```python
from build123d import *

# Parameters (mm, degrees)
ESQUISSE1_W             = 8
ESQUISSE1_H             = 48
BOSS_EXTRU_1_DEPTH      = 45
ESQUISSE28_R            = 7.95
ENL_V_MAT_EXTRU_1_DEPTH = 10
ESQUISSE29_R            = 8.1
ESQUISSE29_R_2          = 5.5
BOSS_EXTRU_2_DEPTH      = 3
ESQUISSE30_R            = 2
ENL_V_MAT_EXTRU_2_DEPTH = 15
ESQUISSE31_R            = 2
ENL_V_MAT_EXTRU_3_DEPTH = 15


with BuildPart() as part:
    # Esquisse1 → Boss.-Extru.1 (new body)
    with BuildSketch(Plane(origin=(0, 0, 0), x_dir=(1, 0, 0), z_dir=(0, 1, 0))):
        with Locations((4, 24)):
            Rectangle(ESQUISSE1_W, ESQUISSE1_H)
    extrude(amount=BOSS_EXTRU_1_DEPTH)

    # Esquisse28 → Enl_v. mat.-Extru.1 (cut)
    with BuildSketch(Plane(origin=(8, 0, 0), x_dir=(0, 0, -1), z_dir=(1, 0, 0))):
        with Locations((24, 18)):
            Circle(ESQUISSE28_R)
    extrude(amount=-ENL_V_MAT_EXTRU_1_DEPTH, mode=Mode.SUBTRACT)

    # Esquisse29 → Boss.-Extru.2 (add)
    with BuildSketch(Plane.ZY):
        with Locations((-24, 18)):
            Circle(ESQUISSE29_R)
        with Locations((-24, 18)):
            Circle(ESQUISSE29_R_2, mode=Mode.SUBTRACT)
    extrude(amount=-BOSS_EXTRU_2_DEPTH)

    # Esquisse30 → Enl_v. mat.-Extru.2 (cut)
    with BuildSketch(Plane.XZ):
        with Locations((4, -44)):
            Circle(ESQUISSE30_R)
        with Locations((4, -4)):
            Circle(ESQUISSE30_R)
    extrude(amount=-ENL_V_MAT_EXTRU_2_DEPTH, mode=Mode.SUBTRACT)

    # Esquisse31 → Enl_v. mat.-Extru.3 (cut)
    with BuildSketch(Plane(origin=(0, 45, 0), x_dir=(1, 0, 0), z_dir=(0, 1, 0))):
        with Locations((4, 44)):
            Circle(ESQUISSE31_R)
        with Locations((4, 4)):
            Circle(ESQUISSE31_R)
    extrude(amount=-ENL_V_MAT_EXTRU_3_DEPTH, mode=Mode.SUBTRACT)


solid = part.part
```
Could you check a few things on this model? Use its own coordinates, in mm. A direction names the side the tool comes from. Coordinates: 2 decimals unless noted, no trailing zeros. Order: outer loops, then holes, each group sorted by start corner. A loop starts at its lowest first (then second) coordinate and runs counter-clockwise, first axis right, second up. Notation, with made-up numbers: M 40.5,-30.75 L 88.5,-30.75 A11 cw 88.5,-15.75 Z; hole C 15,58.25 d10. An arc over 180 degrees is marked long. Use one line per item in the form item = value. Start each with the question number.
1. We'd pull the mould along Z, two halves only. Please class faces 4 (the cylindrical face through (4, 38, -42)), 5 (the flat face through (4, 22, 0)), 6 (the flat face through (0, 27, -24)): +Z half, -Z half, draft (parallel to the pull), parting line (faces both ways), or undercut.
2. Please list where these lines run through material, in increasing order: line 1 (Z direction, x = 4, y = 34.5); line 2 (Z direction, x = 3, y = 42); line 3 (Y direction, x = 1.2, z = -24).
3. Suppose I cut it at A-A on z = -24. Write out the boundary of the cut face in (x, y), then the cut area to 4 significant figures.
4. Suppose I cut it at B-B on x = 4. Write out the boundary of the cut face in (y, z), then the cut area to 3 significant figures.
5. For pin 1 (2 mm diameter, centred on x = 3.5, z = -44, fed in from -Y); pin 2 (6.5 mm diameter, centred on y = 18, z = -24, fed in from -X); pin 3 (2.5 mm diameter, centred on x = 4, z = -44, fed in from +Y), each with a flat end and sliding along its axis, tell me the tip position at first contact or that it passes through.
6. On a 3-axis mill with a long thin cutter (end or side, diameter ignored), from which of +Z, -Z, +X, -X, +Y, -Y can I reach the whole of each face in a straight line? I mean faces 1 (the flat face through (4, 30, -44)), 2 (the flat face through (3, 23.4, -22.3)), 3 (the cylindrical face through (4, 7, -46)). Say none if no direction works.
7. Suppose I cut it at D-D on z = -44. Write out the boundary of the cut face in (x, y), then the cut area to 3 significant figures.
8. Suppose I cut it at C-C on y = 18. Write out the boundary of the cut face in (x, z), then the cut area to 4 significant figures.
Geometry says:
q1.face_4 = undercut
q1.face_5 = +Z half
q1.face_6 = draft
q2.line_1 = -48 to -46, -42 to -6, -2 to 0
q2.line_2 = -48 to -45.73, -42.27 to -5.73, -2.27 to 0
q2.line_3 = 0 to 12.5, 23.5 to 45
q3.outline = M 0,0 L 8,0 L 8,10.05 L 3,10.05 L 3,12.5 L 0,12.5 Z; M 0,23.5 L 3,23.5 L 3,25.95 L 8,25.95 L 8,45 L 0,45 Z
q3.area = 247.5 mm^2
q4.outline = M 0,-48 L 45,-48 L 45,-46 L 30,-46 L 30,-42 L 45,-42 L 45,-6 L 30,-6 L 30,-2 L 45,-2 L 45,0 L 0,0 L 0,-2 L 15,-2 L 15,-6 L 0,-6 L 0,-42 L 15,-42 L 15,-46 L 0,-46 Z; hole C 18,-24 d15.9
q4.area = 1,720 mm^2
q5.pin_1 = 15
q5.pin_2 = through
q5.pin_3 = 30
q6.face_1 = +Y
q6.face_2 = +X
q6.face_3 = -Y
q7.outline = M 0,0 L 2,0 L 2,15 L 6,15 L 6,0 L 8,0 L 8,45 L 6,45 L 6,30 L 2,30 L 2,45 L 0,45 Z
q7.area = 240 mm^2
q8.outline = M 0,-48 L 8,-48 L 8,-31.95 L 3,-31.95 L 3,-29.5 L 0,-29.5 Z; M 0,-18.5 L 3,-18.5 L 3,-16.05 L 8,-16.05 L 8,0 L 0,0 Z
q8.area = 271.5 mm^2
